Here's how the part is built. I have some questions about the finished solid (model axes, mm). A direction names the side the tool comes from. Give positions to 0.01 mm unless a question says otherwise; leave off trailing zeros. Order: outer loops, then holes, each group sorted by start corner. A loop starts at its lowest first (then second) coordinate and runs counter-clockwise, first axis right, second up.
from build123d import *

# Parameters (mm, degrees)
BOSS_EXTRUDE2_DEPTH = 1.5
SKETCH3_W           = 17.792742237
SKETCH3_H           = 21
SKETCH3_W_2         = 18
BOSS_EXTRUDE4_DEPTH = 1
SKETCH5_R           = 5
BOSS_EXTRUDE6_DEPTH = 20.5
FILLET4_R           = 1
CUT_EXTRUDE1_REACH  = 3.5
SKETCH6_R           = 1.5


with BuildPart() as part:
    # Sketch1 → Boss-Extrude2 (new body)
    with BuildSketch(Plane(origin=(0, 0, 0), x_dir=(1, 0, 0), z_dir=(0, 1, 0))):
        with BuildLine():
            Line((-26, 30), (26, 30))
            ThreePointArc((26, 30), (28.121320344, 29.121320344), (29, 27))
            Line((29, 27), (29, -27))
            ThreePointArc((29, -27), (28.121320344, -29.121320344), (26, -30))
            Line((26, -30), (-26, -30))
            ThreePointArc((-26, -30), (-28.121320344, -29.121320344), (-29, -27))
            Line((-29, -27), (-29, 27))
            ThreePointArc((-29, 27), (-28.121320344, 29.121320344), (-26, 30))
        make_face()
    extrude(amount=-BOSS_EXTRUDE2_DEPTH)

    # Sketch3 → Boss-Extrude4 (add)
    with BuildSketch(Plane(origin=(0, 0, 0), x_dir=(1, 0, 0), z_dir=(0, 1, 0))):
        with Locations((15.103628882, 6.5)):
            Rectangle(SKETCH3_W, SKETCH3_H)
        with Locations((-6.792742237, 6.5)):
            Rectangle(SKETCH3_W_2, SKETCH3_H)
    extrude(amount=BOSS_EXTRUDE4_DEPTH)

    # Sketch5 → Boss-Extrude6 (add)
    with BuildSketch(Plane(origin=(0, 0, 0), x_dir=(1, 0, 0), z_dir=(0, 1, 0))):
        with Locations((-16, -10)):
            Circle(SKETCH5_R)
    extrude(amount=BOSS_EXTRUDE6_DEPTH)

    # Fillet4
    fillet4_edges = [part.edges().sort_by_distance(p)[0] for p in [
        (-21, 20.5, 10),
    ]]
    fillet(fillet4_edges, radius=FILLET4_R)

    # Sketch6 → Cut-Extrude1 (cut, up to next)
    with BuildSketch(Plane(origin=(0, 0, 0), x_dir=(1, 0, 0), z_dir=(0, 1, 0)), mode=Mode.PRIVATE) as cut_extrude1_sk1:
        with Locations((-26, 27)):
            Circle(SKETCH6_R)
    cut_extrude1_tool1 = extrude(cut_extrude1_sk1.sketch, amount=-CUT_EXTRUDE1_REACH, mode=Mode.PRIVATE) & part.part
    add(cut_extrude1_tool1.solids().sort_by_distance((-26, 0, -27))[0], mode=Mode.SUBTRACT)
    # Sketch6 → Cut-Extrude1 (cut, up to next)
    with BuildSketch(Plane(origin=(0, 0, 0), x_dir=(1, 0, 0), z_dir=(0, 1, 0)), mode=Mode.PRIVATE) as cut_extrude1_sk2:
        with Locations((26, 27)):
            Circle(SKETCH6_R)
    cut_extrude1_tool2 = extrude(cut_extrude1_sk2.sketch, amount=-CUT_EXTRUDE1_REACH, mode=Mode.PRIVATE) & part.part
    add(cut_extrude1_tool2.solids().sort_by_distance((26, 0, -27))[0], mode=Mode.SUBTRACT)
    # Sketch6 → Cut-Extrude1 (cut, up to next)
    with BuildSketch(Plane(origin=(0, 0, 0), x_dir=(1, 0, 0), z_dir=(0, 1, 0)), mode=Mode.PRIVATE) as cut_extrude1_sk3:
        with Locations((-26, -27)):
            Circle(SKETCH6_R)
    cut_extrude1_tool3 = extrude(cut_extrude1_sk3.sketch, amount=-CUT_EXTRUDE1_REACH, mode=Mode.PRIVATE) & part.part
    add(cut_extrude1_tool3.solids().sort_by_distance((-26, 0, 27))[0], mode=Mode.SUBTRACT)
    # Sketch6 → Cut-Extrude1 (cut, up to next)
    with BuildSketch(Plane(origin=(0, 0, 0), x_dir=(1, 0, 0), z_dir=(0, 1, 0)), mode=Mode.PRIVATE) as cut_extrude1_sk4:
        with Locations((26, -27)):
            Circle(SKETCH6_R)
    cut_extrude1_tool4 = extrude(cut_extrude1_sk4.sketch, amount=-CUT_EXTRUDE1_REACH, mode=Mode.PRIVATE) & part.part
    add(cut_extrude1_tool4.solids().sort_by_distance((26, 0, 27))[0], mode=Mode.SUBTRACT)


solid = part.part
Q1. Thinking about a two-plate mould opening in Z: for faces 1 (the face through (-7, 1, -7)), 2 (the face through (28.14, -0.74, 29.1)), 3 (the face through (25.805, -0.74, -28.487)), which applies, released by +Z, released by -Z, zero draft, split by the parting line, or undercut?
Filled sheet:
face 1: zero draft
face 2: released by +Z
face 3: undercut
Q2. I'm going to push flat-ended pins straight in: P1, Ø12, axis at y = 17, z = 16, coming from the +X side; P2, Ø5.5, axis at x = 17.5, z = -11.5, coming from the +Y side; P3, Ø0.5, axis at x = 18, y = 0.5, coming from the -Z side; P4, Ø1.8, axis at x = 26, z = 27, coming from the +Y side. Where does each tip first touch, or does it pass through?
Filled sheet:
P1: stops at x = -11
P2: stops at y = 1
P3: stops at z = -17
P4: passes through
Q3. If we section it at B-B on z = -3.5: List the corners of the cut face in (x, y) for me, plus the area to 3 significant figures.
Filled sheet:
outline: (-29, -1.5) - (29, -1.5) - (29, 0) - (24, 0) - (24, 1) - (6.21, 1) - (6.21, 0) - (2.21, 0) - (2.21, 1) - (-15.79, 1) - (-15.79, 0) - (-29, 0) - close
area: 123 mm2
Q4. For faces 4 (the face through (-20, 10, 7)), 5 (the face through (-26.195, -0.74, -28.487)), which set-ups out of +Z, -Z, +X, -X, +Y, -Y let a thin tool reach every point of the face, with its end or its side?
Filled sheet:
face 4: +Y
face 5: +Y, -Y
Q5. If we section it at C-C on y = 4: List the corners of the cut face in (x, z) for me, plus the area to 3 significant figures.
Filled sheet:
outline: circle Ø10 at (-16, 10)
area: 78.5 mm2
Q6. If we section it at A-A on x = -7: List the corners of the cut face in (y, z) for me.
Filled sheet:
outline: (-1.5, -30) - (0, -30) - (0, -17) - (1, -17) - (1, 4) - (0, 4) - (0, 30) - (-1.5, 30) - close
Q7. I need wall thicknesses on L1, parallel to Z at x = 26, y = -1; L2, parallel to X at y = -0.8, z = 27; L3, parallel to Y at x = -4, z = 4.5. Which ranges of each line are inside material? Lowest first, please.
Filled sheet:
L1: z = -30 to -28.5, -25.5 to 25.5, 28.5 to 30
L2: x = -29 to -27.5, -24.5 to 24.5, 27.5 to 29
L3: y = -1.5 to 0
